```python
from build123d import *

# Parameters (mm, degrees)
BOSS_EXTRUDE1_DEPTH = 19.05


with BuildPart() as part:
    # Sketch1 → Boss-Extrude1 (new body)
    with BuildSketch(Plane.XY):
        Polygon((3.666174209, -6.35), (7.332348419, 0), (3.666174209, 6.35), (-3.666174209, 6.35), (-7.332348419, 0), (-3.666174209, -6.35), align=None)
        with BuildLine():
            Line((1, 5), (1, 3.872983346))
            ThreePointArc((1, 3.872983346), (3.16227766, 2.449489743), (4, 0))
            ThreePointArc((4, 0), (-2.449489743, -3.16227766), (-1, 3.872983346))
            Line((-1, 3.872983346), (-1, 5))
            Line((-1, 5), (1, 5))
        make_face(mode=Mode.SUBTRACT)
    extrude(amount=BOSS_EXTRUDE1_DEPTH)


solid = part.part
```
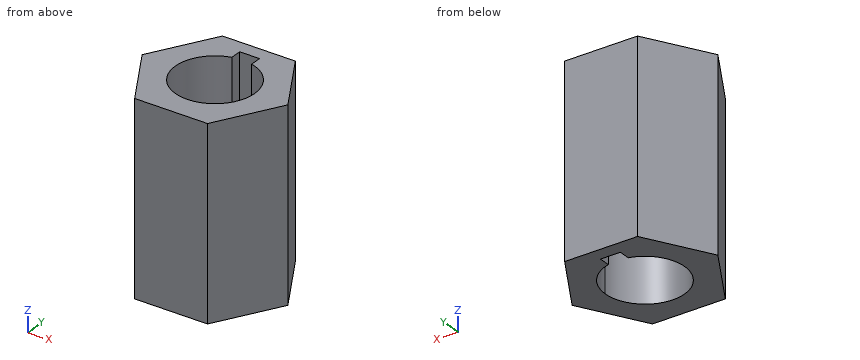
Source: CAD feature listing. Evaluate the final solid. Frame: model axes, mm. Coordinates: 2 decimals unless noted, no trailing zeros. Loops run counter-clockwise (first coordinate to the right, second up) from the corner with the lowest first, then second, coordinate; pieces in that order, holes last. Notation, with made-up numbers: M -2,20.25 L 32,20.25 A21 cw 32,42.25 Z; hole C 64,14 d11. An arc over 180 degrees is marked long. Use a Markdown table: item, result. Add a question column.
Q1. Section query B-B, the plane z = 10. Return loops of the section in (x, y).
Q2. Section query A-A, the plane x = 0. Return loops of the section in (y, z).
Q3. Section query D-D, the plane x = 5.75. Return loops of the section in (y, z).
Q4. First-contact query: pin 1 (6 mm diameter, centred on y = 2.5, z = 10.5, fed in from -X); pin 2 (0.9 mm diameter, centred on y = 4.5, z = 10.5, fed in from -X); pin 3 (5 mm diameter, centred on y = 5, z = 2.5, fed in from -X). Flat tips, straight axial feed; report the tip coordinate or a pass-through.
Q5. Material intervals for L1, parallel to Y at x = 0, z = 7.75; L2, parallel to Y at x = -1.5, z = 8; L3, parallel to X at y = 2.75, z = 3.5, sorted ascending.
Q6. Section query C-C, the plane y = -3.5. Return loops of the section in (x, z), and give its area (3 significant figures).
Result:
| question | item | result |
|---|---|---|
| 1 | outline | M -7.33,0 L -3.67,-6.35 L 3.67,-6.35 L 7.33,0 L 3.67,6.35 L -3.67,6.35 Z; hole M -1,3.87 A4 ccw long 1,3.87 L 1,5 L -1,5 Z |
| 2 | outline | M -6.35,0 L -4,0 L -4,19.05 L -6.35,19.05 Z; M 5,0 L 6.35,0 L 6.35,19.05 L 5,19.05 Z |
| 3 | outline | M -2.74,0 L 2.74,0 L 2.74,19.05 L -2.74,19.05 Z |
| 4 | pin 1 | stops at x = -7.33 |
| 4 | pin 2 | stops at x = -4.99 |
| 4 | pin 3 | stops at x = -5.89 |
| 5 | L1 | y = -6.35 to -4, 5 to 6.35 |
| 5 | L2 | y = -6.35 to -3.71, 3.71 to 6.35 |
| 5 | L3 | x = -5.74 to -2.9, 2.9 to 5.74 |
| 6 | outline | M -5.31,0 L -1.94,0 L -1.94,19.05 L -5.31,19.05 Z; M 1.94,0 L 5.31,0 L 5.31,19.05 L 1.94,19.05 Z |
| 6 | area | 129 mm2 |
